Source: CAD feature listing. Evaluate the final solid. Frame: model axes, mm. Give positions to 0.01 mm unless a question says otherwise; leave off trailing zeros. Loops run counter-clockwise (first coordinate to the right, second up) from the corner with the lowest first, then second, coordinate; pieces in that order, holes last. Notation, with made-up numbers: M 67,7.25 L 108,7.25 A35 ccw 108,42.25 Z; hole C 31.25,62 d8. An arc over 180 degrees is marked long. Answer in a Markdown table with one row per item.
```python
from build123d import *

# Parameters (mm, degrees)
SLIDER_MAIN_BODY_DEPTH = 5
SKETCH4_W              = 105.16
SKETCH4_H              = 1.666666666
CUT_EXTRUDE1_DEPTH     = 64.492125496


with BuildPart() as part:
    # Sketch1 → Slider Main Body (new body)
    with BuildSketch(Plane.XY):
        Polygon((-57.58, 7.5), (-57.58, 2.5), (57.58, 2.5), (57.58, 7.5), (62.5, 7.5), (62.5, -7.5), (57.58, -7.5), (57.58, -2.5), (-57.58, -2.5), (-57.58, -7.5), (-62.5, -7.5), (-62.5, 7.5), align=None)
    extrude(amount=SLIDER_MAIN_BODY_DEPTH)

    # Sketch4 → Cut-Extrude1 (cut, through all)
    with BuildSketch(Plane.XZ.offset(2.5)):
        with Locations((0, 2.5)):
            Rectangle(SKETCH4_W, SKETCH4_H)
    extrude(amount=-CUT_EXTRUDE1_DEPTH, mode=Mode.SUBTRACT)


solid = part.part
```
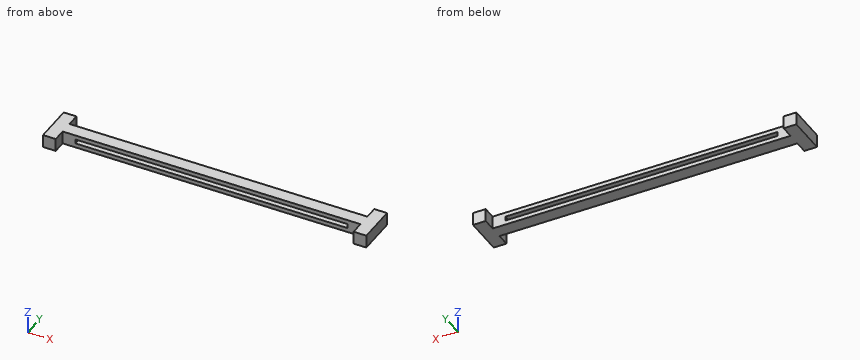
Q1. Ray query, probe 1 along X at (y, z) = (-4.5, 1.9); probe 2 along Z at (x, y) = (31.5, 0.5); probe 3 along X at (y, z) = (-0.75, 2.2). Return the intervals inside material, ascending. Write a range as from..to.
Values follow:
| item | result |
|---|---|
| probe 1 | -62.5..-57.58, 57.58..62.5 |
| probe 2 | 0..1.67, 3.33..5 |
| probe 3 | -62.5..-52.58, 52.58..62.5 |
Q2. Section query A-A (x = 34.5). Output: boundary loops of the cut face in (y, z), plus the area to 3 significant figures.
Values follow:
| item | result |
|---|---|
| outline | M -2.5,0 L 2.5,0 L 2.5,1.67 L -2.5,1.67 Z; M -2.5,3.33 L 2.5,3.33 L 2.5,5 L -2.5,5 Z |
| area | 16.7 mm^2 |
Q3. Section query B-B (y = 0.5). Output: boundary loops of the cut face in (x, z), plus the area to 3 significant figures.
Values follow:
| item | result |
|---|---|
| outline | M -62.5,0 L 62.5,0 L 62.5,5 L -62.5,5 Z; hole M -52.58,1.67 L 52.58,1.67 L 52.58,3.33 L -52.58,3.33 Z |
| area | 450 mm^2 |
